Verification items for the finished model (mm, model axes). A direction names the side the tool comes from. Coordinates: 2 decimals unless noted, no trailing zeros. Write each loop counter-clockwise with the first axis right and the second up, starting at its lowest first coordinate (ties: lowest second). Pieces come first, ordered by that corner, then holes. Notation, with made-up numbers: (6, 60.25) -> (29, 60.25) arc R20 ccw to (29, 81.25) -> close; hole circle Ø10 at (-12, 57.5). An arc over 180 degrees is marked (long way). Answer in a Markdown table with one row per item.
```python
from build123d import *

# Parameters (mm, degrees)
BOX190_W                   = 38
BOX190_H                   = 20
BOX190_DEPTH               = 12.5
BOX190_PLACEMENT_ANGLE     = 3
BOX180_W                   = 20
BOX180_H                   = 10
BOX180_DEPTH               = 18
CYLINDER195_R              = 1.25
CYLINDER195_DEPTH          = 10
CYLINDER194_R              = 1.25
CYLINDER194_DEPTH          = 10
BOX106_W                   = 12
BOX106_H                   = 20
BOX106_DEPTH               = 12.5
BOX105_W                   = 12.5
BOX105_H                   = 12.5
BOX105_DEPTH               = 60
BOX104_W                   = 18
BOX104_H                   = 16
BOX104_DEPTH               = 65
CHAMFER014_SIZE            = 1.1
CHAMFER014_PLACEMENT_ANGLE = 3
CYLINDER246_R              = 1.6
CYLINDER246_DEPTH          = 10
BOX189_W                   = 7.5
BOX189_H                   = 3
BOX189_DEPTH               = 7
FILLET071_R                = 3
CYLINDER244_R              = 1.6
CYLINDER244_DEPTH          = 10
CYLINDER245_R              = 3.1
CYLINDER245_DEPTH          = 10
CYLINDER247_R              = 3.1
CYLINDER247_DEPTH          = 10
CYLINDER248_R              = 1.6
CYLINDER248_DEPTH          = 10
BOX188_W                   = 50
BOX188_H                   = 10
BOX188_DEPTH               = 11
BOX187_W                   = 18
BOX187_H                   = 10
BOX187_DEPTH               = 11
BOX187_PLACEMENT_ANGLE     = 3
CHAMFER016_SIZE            = 9


with BuildPart() as cube277:
    # Box190 → Box190 (new body)
    with BuildSketch(Plane.XY):
        with Locations((19, 10)):
            Rectangle(BOX190_W, BOX190_H)
    extrude(amount=BOX190_DEPTH)


with BuildPart() as cube277_1:
    # Box190 placement: moved
    add(cube277.part.moved(Location((223, -16, 15.7))).rotate(Axis((223, -16, 15.7), (0, -1, 0)), BOX190_PLACEMENT_ANGLE))


with BuildPart() as cube267:
    # Box180 → Box180 (new body)
    with BuildSketch(Plane(origin=(231, 0, -7), x_dir=(1, 0, 0), z_dir=(0, 0, 1))):
        with Locations((10, 5)):
            Rectangle(BOX180_W, BOX180_H)
    extrude(amount=BOX180_DEPTH)


with BuildPart() as cylinder482:
    # Cylinder195 → Cylinder195 (new body)
    with BuildSketch(Plane(origin=(323, 0, -39), x_dir=(0, 0, -1), z_dir=(1, 0, 0))):
        Circle(CYLINDER195_R)
    extrude(amount=CYLINDER195_DEPTH)


with BuildPart() as fusion167:
    # Cylinder194 → Cylinder194 (new body)
    with BuildSketch(Plane(origin=(323, 0, -59), x_dir=(0, 0, -1), z_dir=(1, 0, 0))):
        Circle(CYLINDER194_R)
    extrude(amount=CYLINDER194_DEPTH)

    # Fusion167: union Cylinder482
    add(cylinder482.part)


with BuildPart() as fusion167_1:
    # Fusion167 placement: moved
    add(fusion167.part.moved(Location((40, 2, 0))))


with BuildPart() as cube174:
    # Box106 → Box106 (new body)
    with BuildSketch(Plane(origin=(363.75, -10, -55.25), x_dir=(1, 0, 0), z_dir=(0, 0, 1))):
        with Locations((6, 10)):
            Rectangle(BOX106_W, BOX106_H)
    extrude(amount=BOX106_DEPTH)


with BuildPart() as cube173:
    # Box105 → Box105 (new body)
    with BuildSketch(Plane(origin=(353.75, -4.25, -65), x_dir=(1, 0, 0), z_dir=(0, 0, 1))):
        with Locations((6.25, 6.25)):
            Rectangle(BOX105_W, BOX105_H)
    extrude(amount=BOX105_DEPTH)


with BuildPart() as cut190:
    # Box104 → Box104 (new body)
    with BuildSketch(Plane(origin=(352, -6, -65), x_dir=(1, 0, 0), z_dir=(0, 0, 1))):
        with Locations((9, 8)):
            Rectangle(BOX104_W, BOX104_H)
    extrude(amount=BOX104_DEPTH)

    # Cut125: cut Cube173
    add(cube173.part, mode=Mode.SUBTRACT)

    # Cut124: cut Cube174
    add(cube174.part, mode=Mode.SUBTRACT)

    # Cut187: cut Fusion167
    add(fusion167_1.part, mode=Mode.SUBTRACT)


with BuildPart() as cut190_1:
    # Cut187 placement: moved
    add(cut190.part.moved(Location((-120, -9, 10))))

    # Chamfer014
    chamfer014_edges = [cut190_1.edges().sort_by_distance(p)[0] for p in [
        (246.25, -7, -45.25),
        (246.25, -7, -32.75),
    ]]
    chamfer(chamfer014_edges, length=CHAMFER014_SIZE)


with BuildPart() as cut190_2:
    # Chamfer014 placement: moved
    add(cut190_1.part.moved(Location((0, 0, -13))).rotate(Axis((0, 0, -13), (0, -1, 0)), CHAMFER014_PLACEMENT_ANGLE))

    # Cut190: cut Cube267
    add(cube267.part, mode=Mode.SUBTRACT)


with BuildPart() as cut190_3:
    # Cut190 placement: moved
    add(cut190_2.part.moved(Location((0, 0, 7))))


with BuildPart() as cylinder530:
    # Cylinder246 → Cylinder246 (new body)
    with BuildSketch(Plane(origin=(253, 7, 6.5), x_dir=(1, 0, 0), z_dir=(0, -1, 0))):
        Circle(CYLINDER246_R)
    extrude(amount=CYLINDER246_DEPTH)


with BuildPart() as fillet071:
    # Box189 → Box189 (new body)
    with BuildSketch(Plane(origin=(249, -3, 3), x_dir=(1, 0, 0), z_dir=(0, 0, 1))):
        with Locations((3.75, 1.5)):
            Rectangle(BOX189_W, BOX189_H)
    extrude(amount=BOX189_DEPTH)

    # Cut196: cut Cylinder530
    add(cylinder530.part, mode=Mode.SUBTRACT)

    # Fillet071
    fillet071_edges = [fillet071.edges().sort_by_distance(p)[0] for p in [
        (256.5, -1.5, 10),
        (256.5, -1.5, 3),
    ]]
    fillet(fillet071_edges, radius=FILLET071_R)


with BuildPart() as fillet071_1:
    # Fillet071 placement: moved
    add(fillet071.part.moved(Location((-0.5, 0, 0.5))))


with BuildPart() as cylinder528:
    # Cylinder244 → Cylinder244 (new body)
    with BuildSketch(Plane(origin=(246, 6, -9), x_dir=(1, 0, 0), z_dir=(0, 0, 1))):
        Circle(CYLINDER244_R)
    extrude(amount=CYLINDER244_DEPTH)


with BuildPart() as cylinder529:
    # Cylinder245 → Cylinder245 (new body)
    with BuildSketch(Plane(origin=(246, 6, -12), x_dir=(1, 0, 0), z_dir=(0, 0, 1))):
        Circle(CYLINDER245_R)
    extrude(amount=CYLINDER245_DEPTH)


with BuildPart() as cylinder531:
    # Cylinder247 → Cylinder247 (new body)
    with BuildSketch(Plane(origin=(236, 6, -12), x_dir=(1, 0, 0), z_dir=(0, 0, 1))):
        Circle(CYLINDER247_R)
    extrude(amount=CYLINDER247_DEPTH)


with BuildPart() as fusion209:
    # Cylinder248 → Cylinder248 (new body)
    with BuildSketch(Plane(origin=(236, 6, -9), x_dir=(1, 0, 0), z_dir=(0, 0, 1))):
        Circle(CYLINDER248_R)
    extrude(amount=CYLINDER248_DEPTH)

    # Fusion209: union Cylinder528, Cylinder529, Cylinder531
    add(cylinder528.part)
    add(cylinder529.part)
    add(cylinder531.part)


with BuildPart() as fusion209_1:
    # Fusion209 placement: moved
    add(fusion209.part.moved(Location((0, 0, -1))))


with BuildPart() as cube275:
    # Box188 → Box188 (new body)
    with BuildSketch(Plane(origin=(231, 0, 0), x_dir=(1, 0, 0), z_dir=(0, 0, 1))):
        with Locations((25, 5)):
            Rectangle(BOX188_W, BOX188_H)
    extrude(amount=BOX188_DEPTH)


with BuildPart() as supports_left_frame:
    # Box187 → Box187 (new body)
    with BuildSketch(Plane.XY):
        with Locations((9, 5)):
            Rectangle(BOX187_W, BOX187_H)
    extrude(amount=BOX187_DEPTH)


with BuildPart() as supports_left_frame_1:
    # Box187 placement: moved
    add(supports_left_frame.part.moved(Location((232.21, 0, -11))).rotate(Axis((232.21, 0, -11), (0, -1, 0)), BOX187_PLACEMENT_ANGLE))

    # Cut194: cut Cube275
    add(cube275.part, mode=Mode.SUBTRACT)

    # Chamfer016
    chamfer016_edges = [supports_left_frame_1.edges().sort_by_distance(p)[0] for p in [
        (241.197666, 10, -10.528976),
    ]]
    chamfer(chamfer016_edges, length=CHAMFER016_SIZE)

    # Cut195: cut Fusion209
    add(fusion209_1.part, mode=Mode.SUBTRACT)


with BuildPart() as supports_left_frame_2:
    # Cut195 placement: moved
    add(supports_left_frame_1.part.moved(Location((0.371, 0, 0))))

    # Fusion213: union Cut190, Fillet071
    add(cut190_3.part)
    add(fillet071_1.part)

    # Cut197: cut Cube277
    add(cube277_1.part, mode=Mode.SUBTRACT)


with BuildPart() as supports_left_frame_3:
    # Cut197 placement: moved
    add(supports_left_frame_2.part.moved(Location((0, -10, 0))))


solid = supports_left_frame_3.part
```
1. Material ranges on probe 1 along X at (y, z) = (-4, -1.3); probe 2 along Y at (x, z) = (241, -21); probe 3 along X at (y, z) = (-4, -0.8), recorded low to high. Write a range as from..to.
Findings below:
| item | result |
|---|---|
| probe 1 | x = 232.07..234.77, 237.97..244.77, 247.97..250.1 |
| probe 2 | y = -25..-23.25, -10.75..-9 |
| probe 3 | x = 232.05..234.77, 237.97..244.77, 247.97..250.07 |
2. Sectioned sample at C-C, the plane z = 9.5. Record the cut outline in (x, y), and give its area (3 significant figures).
Findings below:
| item | result |
|---|---|
| outline | (231.51, -25) -> (249.53, -25) -> (249.53, -13) -> (255.24, -13) -> (255.24, -10) -> (231.51, -10) -> close; hole (233.26, -23.25) -> (245.78, -23.25) -> (245.78, -10.75) -> (233.26, -10.75) -> close |
| area | 131 mm² |
3. Access from +Z, -Z, +X, -X, +Y, -Y to the whole of each face (thin tool, end or side, straight path). Record for faces 4 (the face through (247, -6, -3)), 5 (the face through (245.19, -2.92, -1.52)), 6 (the face through (251, -11, 10.5)), 7 (the face through (241, -23.25, -19)), 8 (the face through (241, -5, 0)).
Findings below:
| item | result |
|---|---|
| face 4 | -Z |
| face 5 | +Z, -Z |
| face 6 | +Z, +X, +Y, -Y |
| face 7 | none |
| face 8 | +Z, +X, -X, +Y |
4. Sectioned sample at A-A, the plane y = -4. Record the cut outline in (x, z).
Findings below:
| item | result |
|---|---|
| outline | (232.01, -0.02) -> (232.32, -6.01) -> (233.27, -5.96) -> (233.27, -3) -> (234.77, -3) -> (234.77, 0) -> (232.29, 0) -> close; (237.97, -3) -> (239.47, -3) -> (239.47, -5.63) -> (243.27, -5.43) -> (243.27, -3) -> (244.77, -3) -> (244.77, 0) -> (237.97, 0) -> close; (247.97, -3) -> (249.47, -3) -> (249.47, -5.11) -> (250.29, -5.06) -> (250.03, 0) -> (247.97, 0) -> close |
5. Sectioned sample at B-B, the plane z = -12. Record the cut outline in (x, y).
Findings below:
| item | result |
|---|---|
| outline | (232.63, -25) -> (250.66, -25) -> (250.66, -9) -> (232.63, -9) -> close; hole (234.39, -23.25) -> (246.9, -23.25) -> (246.9, -10.75) -> (234.39, -10.75) -> close |
6. Go/stop test with flat-tipped pins: pin 1 (7 mm diameter, centred on x = 236.371, y = -4, fed in from +Z); pin 2 (2.5 mm diameter, centred on x = 252.5, z = 7, fed in from +Y); pin 3 (3 mm diameter, centred on y = -14.5, z = -14.5, fed in from -X); pin 4 (6 mm diameter, centred on x = 245.5, y = -5.5, fed in from -Z). Record where each tip stops, or that it passes through.
Findings below:
| item | result |
|---|---|
| pin 1 | stops at z = 0 |
| pin 2 | passes through |
| pin 3 | stops at x = 232.69 |
| pin 4 | stops at z = -9.83 |
7. Release check for a two-part mould opening along X. For faces 1 (the face through (242, -9, -30)), 2 (the face through (246.623, -17.088, -6.675)), 3 (the face through (255.1, -11.48, 4.36)) record: released by +X, released by -X, zero draft, split by the parting line, or undercut.
Findings below:
| item | result |
|---|---|
| face 1 | zero draft |
| face 2 | undercut |
| face 3 | released by +X |
